Here's how the part is built. I have some questions about the finished solid (model axes, mm). Face numbers are marked on the shaded views. Coordinates: 2 decimals unless noted, no trailing zeros. Write each loop counter-clockwise with the first axis right and the second up, starting at its lowest first coordinate (ties: lowest second). Pieces come first, ordered by that corner, then holes.
```python
from build123d import *

# Parameters (mm, degrees)
CROQUIS1_R              = 1.5
SALIENTE_EXTRUIR1_DEPTH = 2
REDONDEO1_R             = 5


with BuildPart() as part:
    # Croquis1 → Saliente-Extruir1 (new body)
    with BuildSketch(Plane(origin=(0, 0, 0), x_dir=(1, 0, 0), z_dir=(0, 1, 0))):
        Polygon((-13, 0), (-13, 5), (0, 5), (18.5, 5), (25, 2.5), (25, 0), (25, -2.5), (18.5, -5), (0, -5), (-13, -5), align=None)
        with Locations(Location((-9.5, 0, 0), (0, 0, 270))):
            Circle(CROQUIS1_R, mode=Mode.SUBTRACT)
    extrude(amount=SALIENTE_EXTRUIR1_DEPTH)

    # Redondeo1
    redondeo1_edges = [part.edges().sort_by_distance(p)[0] for p in [
        (-13, 1, 5),
        (-13, 1, -5),
    ]]
    fillet(redondeo1_edges, radius=REDONDEO1_R - 0.0001)  # a hair under: the kernel refuses the full size


solid = part.part
```
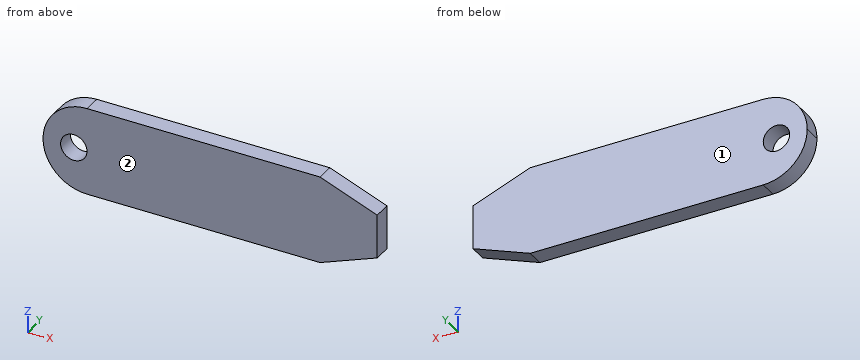
1) Imagine slicing it at D-D on z = -3.75. Please give me the cut outline in (x, y).
Values follow:
outline: (-11.31, 0) - (21.75, 0) - (21.75, 2) - (-11.31, 2) - close
2) I need wall thicknesses on probe 1 along X at (y, z) = (0.8, 0); probe 2 along X at (y, z) = (1.7, 1); probe 3 along Z at (x, y) = (23, 1.1). Which ranges of each line are inside material? Lowest first, please.
Values follow:
probe 1: x = -13 to -11, -8 to 25
probe 2: x = -12.9 to -10.62, -8.38 to 25
probe 3: z = -3.27 to 3.27
3) Imagine slicing it at C-C on z = -1. Please give me the cut outline in (x, y).
Values follow:
outline: (-12.9, 0) - (-10.62, 0) - (-10.62, 2) - (-12.9, 2) - close; (-8.38, 0) - (25, 0) - (25, 2) - (-8.38, 2) - close
4) We'd pull the mould along Y, two halves only. Please class the marked faces 1 and 2: pulls with the +Y half, pulls with the -Y half, needs draft (parallel to the pull), parting line crosses it, or undercut.
Values follow:
face 1: pulls with the +Y half
face 2: pulls with the -Y half
5) Imagine slicing it at B-B on x = -10. Please give me the cut outline in (y, z), then the cut area to 3 significant figures.
Values follow:
outline: (0, -4.58) - (2, -4.58) - (2, -1.41) - (0, -1.41) - close; (0, 1.41) - (2, 1.41) - (2, 4.58) - (0, 4.58) - close
area: 12.7 mm2
